Autodesk Inventor part; units mm, degrees
ref_plane "YZ Plane" through (0, 0, 0) normal (1, 0, 0) x (0, 1, 0)
ref_plane "XZ Plane" through (0, 0, 0) normal (0, 1, 0) x (-1, 0, 0)
ref_plane "XY Plane" through (0, 0, 0) normal (0, 0, 1) x (1, 0, 0)
sketch "Sketch2" plane through (0, 0, 0) normal (0, 0, 1) x (1, 0, 0)
  line L0 (0, 0) -> (0, -42.7)
  line L1 (0, 0) -> (-8, 0)
  line L2 (-8, 0) -> (-8, -3.7)
  line L3 (-8, -3.7) -> (0, -3.7)
  line L4 (0, -3.7) -> (0, 0)
  line L5 (0, -3.7) -> (-6, -3.7)
  line L6 (-6, -3.7) -> (-6, -9.7)
  line L7 (-6, -9.7) -> (0, -9.7)
  line L8 (0, -9.7) -> (0, -3.7)
  line L9 (0, -9.7) -> (-8, -9.7)
  line L10 (-8, -9.7) -> (-8, -12.7)
  line L11 (-8, -12.7) -> (0, -12.7)
  line L12 (0, -12.7) -> (0, -9.7)
  line L13 (0, -42.7) -> (-11.15, -42.7)
  line L14 (-11.15, -42.7) -> (-11.15, -41.7)
  line L15 (-11.15, -41.7) -> (0, -41.7)
  line L16 (0, -41.7) -> (0, -42.7)
  line L17 (-11.15, -39.2) -> (0, -39.2)
  line L18 (0, -39.2) -> (0, -40.2)
  line L19 (0, -40.2) -> (-11.15, -40.2)
  line L20 (-11.15, -40.2) -> (-11.15, -39.2)
  line L21 (-11.15, -36.7) -> (0, -36.7)
  line L22 (0, -36.7) -> (0, -37.7)
  line L23 (0, -37.7) -> (-11.15, -37.7)
  line L24 (-11.15, -37.7) -> (-11.15, -36.7)
  line L25 (-11.15, -34.2) -> (0, -34.2)
  line L26 (0, -34.2) -> (0, -35.2)
  line L27 (0, -35.2) -> (-11.15, -35.2)
  line L28 (-11.15, -35.2) -> (-11.15, -34.2)
  line L29 (-11.15, -31.7) -> (0, -31.7)
  line L30 (0, -31.7) -> (0, -32.7)
  line L31 (0, -32.7) -> (-11.15, -32.7)
  line L32 (-11.15, -32.7) -> (-11.15, -31.7)
  line L33 (-11.15, -29.2) -> (0, -29.2)
  line L34 (0, -29.2) -> (0, -30.2)
  line L35 (0, -30.2) -> (-11.15, -30.2)
  line L36 (-11.15, -30.2) -> (-11.15, -29.2)
  line L37 (-11.15, -26.7) -> (0, -26.7)
  line L38 (0, -26.7) -> (0, -27.7)
  line L39 (0, -27.7) -> (-11.15, -27.7)
  line L40 (-11.15, -27.7) -> (-11.15, -26.7)
  line L41 (-11.15, -24.2) -> (0, -24.2)
  line L42 (0, -24.2) -> (0, -25.2)
  line L43 (0, -25.2) -> (-11.15, -25.2)
  line L44 (-11.15, -25.2) -> (-11.15, -24.2)
  line L45 (-11.15, -21.7) -> (0, -21.7)
  line L46 (0, -21.7) -> (0, -22.7)
  line L47 (0, -22.7) -> (-11.15, -22.7)
  line L48 (-11.15, -22.7) -> (-11.15, -21.7)
  line L49 (-11.15, -19.2) -> (0, -19.2)
  line L50 (0, -19.2) -> (0, -20.2)
  line L51 (0, -20.2) -> (-11.15, -20.2)
  line L52 (-11.15, -20.2) -> (-11.15, -19.2)
  line L53 (-11.15, -16.7) -> (0, -16.7)
  line L54 (0, -16.7) -> (0, -17.7)
  line L55 (0, -17.7) -> (-11.15, -17.7)
  line L56 (-11.15, -17.7) -> (-11.15, -16.7)
  line L57 (0, -14.2) -> (-8, -14.2)
  line L58 (-8, -14.2) -> (-8, -15.2)
  line L59 (-8, -15.2) -> (0, -15.2)
  line L60 (0, -15.2) -> (0, -14.2)
  line L61 (0, -12.7) -> (0, -39.2)
  line L62 (-4, -15.2) -> (-4, -16.7)
  line L63 (-4, -14.2) -> (-4, -12.7)
  line L64 (-4, -16.7) -> (-6, -41.7)
  line L65 (-4.2, -17.7) -> (-4.2, -19.2)
  line L66 (-4.4, -21.7) -> (-4.4, -20.2)
  line L67 (-4.6, -24.2) -> (-4.6, -22.7)
  line L68 (-4.8, -26.7) -> (-4.8, -25.2)
  line L69 (-5, -29.2) -> (-5, -27.7)
  line L70 (-5.2, -31.7) -> (-5.2, -30.2)
  line L71 (-5.4, -34.2) -> (-5.4, -32.7)
  line L72 (-5.6, -36.7) -> (-5.6, -35.2)
  line L73 (-5.8, -39.2) -> (-5.8, -37.7)
  line L74 (-6, -41.7) -> (-6, -40.2)
  line L75 (0, -17.7) -> (0, -41.7)
  line L76 (0, -12.7) -> (0, -14.2)
  line L77 (0, -15.2) -> (0, -16.7)
  line L78 (0, -30.2) -> (0, -31.7)
  line L79 (0, -42.7) -> (-2, -42.7)
  line L80 (-2, -42.7) -> (-2, -49.8)
  line L81 (-2, -49.8) -> (0, -49.8)
  line L82 (0, -49.8) -> (0, -42.7)
  line L83 (0, -49.8) -> (-3, -49.8)
  line L84 (-3, -49.8) -> (-3, -55.8)
  line L85 (-3, -55.8) -> (0, -55.8)
  line L86 (0, -55.8) -> (0, -49.8)
  line L87 (0, -55.8) -> (-2.5, -55.8)
  line L88 (-2.5, -55.8) -> (-2.5, -57.3)
  line L89 (-2.5, -57.3) -> (0, -57.3)
  line L90 (0, -57.3) -> (0, -55.8)
  line L91 (0, -57.3) -> (-3.5, -57.3)
  line L92 (-3.5, -57.3) -> (-3.5, -60.3)
  line L93 (-3.5, -60.3) -> (0, -60.3)
  line L94 (0, -60.3) -> (0, -57.3)
  line L95 (-1.9004, -60.3) -> (-0.5, -62.3)
  line L96 (-0.5, -62.3) -> (0, -62.3)
  line L97 (0, -62.3) -> (0, -60.3)
  dimension "d21" = 42.7
  dimension "d22" = 8
  dimension "d23" = 3.7
  dimension "d24" = 6
  dimension "d25" = 6
  dimension "d26" = 8
  dimension "d27" = 3
  dimension "d28" = 11.15
  dimension "d29" = 1
  dimension "d39" = 2.5
  dimension "d44" = 8
  dimension "d45" = 1
  dimension "d46" = 1.5
  dimension "d48" = 12
  dimension "d50" = 2
  dimension "d51" = 7.1
  dimension "d52" = 3
  dimension "d53" = 6
  dimension "d54" = 2.5
  dimension "d55" = 1.5
  dimension "d56" = 3.5
  dimension "d57" = 10.5
  dimension "d58" = 125
  dimension "d59" = 0.5
  dimension "d60" = 2
revolve "Revolution1" add sketch "Sketch2" angle 360 about axis through (0, -31.7, 0) along (0, -1, 0)
sketch "Sketch3" plane through (0, -60.3, 0) normal (0, -1, 0) x (1, 0, 0)
  circle A0 centre (0, 0) radius 3.5
  circle A1 centre (0, 0) radius 1.9004
  line L0 (4.0415, 0) -> (2.0207, -3.5)
  line L1 (2.0207, -3.5) -> (-2.0207, -3.5)
  line L2 (-2.0207, -3.5) -> (-4.0415, 0)
  line L3 (-4.0415, 0) -> (-2.0207, 3.5)
  line L4 (-2.0207, 3.5) -> (2.0207, 3.5)
  line L5 (2.0207, 3.5) -> (4.0415, 0)
  circle A2 centre (0, 0) radius 12.5
  dimension "d61" = 7
  dimension "d62" = 25
extrude "Extrusion1" add sketch "Sketch3" against normal up to surface (3 mm away) contours A0 L5 L0 | A0 L4 L5 | L0 L1 A0 | A0 L3 L4 | L1 L2 A0 | A0 L2 L3
sketch "Sketch4" plane through (0, 0, 0) normal (1, 0, 0) x (0, 1, 0)
  line L0 (-45.05, 15.5) -> (-56.55, 15.5)
  line L1 (-56.55, 15.5) -> (-56.55, -4.5)
  line L2 (-56.55, -4.5) -> (-45.05, -4.5)
  line L3 (-45.05, -4.5) -> (-45.05, 15.5)
  arc A0 (-53.05, 9.9834) -> (-52.05, 9.9834) centre (-52.55, 7) ccw
  line L4 (-60.3, 0) -> (-57.3, 0)
  line L5 (-52.55, 7) -> (-52.55, 15.5) construction
  line L6 (-53.05, 15.5) -> (-53.05, 9.9834)
  line L7 (-52.05, 9.9834) -> (-52.05, 15.5)
  line L8 (-57.3, 2.5) -> (-55.8, 2.5)
  point P0 (0, 0)
  point P1 (-52.55, 11.25)
  point P2 (-56.55, 2.5)
  dimension "d65" = 11.5
  dimension "d66" = 20
  dimension "d67" = 6.05
  dimension "d68" = 4
  dimension "d69" = 11.5
  dimension "d70" = 4.5
  dimension "d84" = 3.5
  dimension "d85" = 4.5
extrude "Extrusion2" add sketch "Sketch4" along normal mid plane 16 contours L3 L2 L1 L0 L6 A0 L7
sketch "Sketch5" plane through (0, -62.3, 0) normal (0, -1, 0) x (1, 0, 0)
  circle A0 centre (0, 0) radius 0.2
  dimension "d75" = 0.4
extrude "Extrusion3" cut sketch "Sketch5" against normal through all
sketch "Sketch6" plane through (0, 0, 0) normal (0, 1, 0) x (1, 0, 0)
  circle A0 centre (0, 0) radius 1
  dimension "d78" = 2
extrude "Extrusion4" cut sketch "Sketch6" against normal up to surface (60.3 mm away)
chamfer "Chamfer1" distance 1 angle 45 1 edges at (-1, 0, 0)
chamfer "Chamfer2" distance 0.5 angle 45 14 edges at (-8, -56.55, 5.5) (0, -56.55, 15.5) (-8, -54.8, 15.5) (-8, -48.55, 15.5) (8, -48.55, 15.5) (0, -45.05, 15.5) (-8, -45.05, 5.5) (-8, -50.8, -4.5) (0, -56.55, -4.5) (8, -56.55, 5.5) (8, -50.8, -4.5) (8, -45.05, 5.5) (8, -54.8, 15.5) (0, -45.05, -4.5)
sketch "Sketch7" plane through (0, 0, 0) normal (0, 0, 1) x (1, 0, 0)
  line L0 (-4.0415, -60.3) -> (-2.0207, -60.3)
  line L1 (-4.0415, -60.3) -> (-4.0415, -57.3)
  line L2 (-4.0415, -60.05) -> (-3.7915, -60.3)
  line L3 (0, -74.76) -> (0, 12.46)
  line L4 (-2.0207, -57.3) -> (-4.0415, -57.3)
  line L5 (-4.0415, -57.55) -> (-3.7915, -57.3)
  point P0 (0, 0)
  dimension "d89" = 0.25
  dimension "d90" = 0.25
  dimension "d92" = 0.25
  dimension "d93" = 0.25
revolve "Revolution2" cut sketch "Sketch7" angle 360 about axis through (0, -10, 0) along (0, 1, 0)
equation "\"d90\" = d89"
equation "\"d92\" = d89"
equation "\"d93\" = d89"
properties part number "e3dv6"
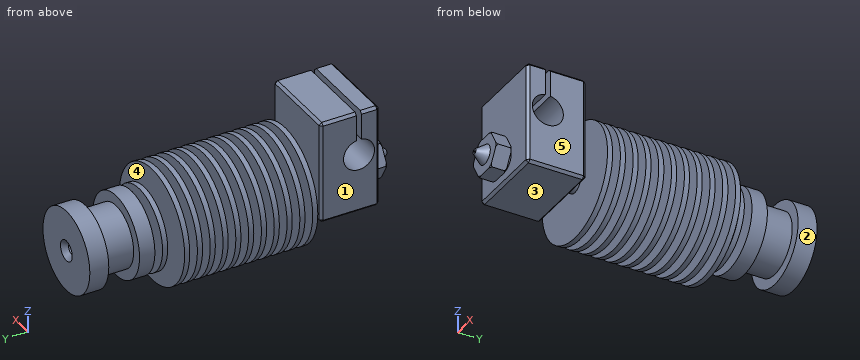
Geometry: final body of the model. Coordinates: model frame, mm. Face numbers are marked on the shaded views. A direction names the side the tool comes from. Round coordinates to 2 decimals unless told otherwise and drop trailing zeros. Order: outer loops, then holes, each group sorted by start corner. A loop starts at its lowest first (then second) coordinate and runs counter-clockwise, first axis right, second up. Notation, with made-up numbers: (37.25, -25) - (94.25, -25) arc R32 ccw to (94.25, 7) - close; hole circle Ø9 at (39, 59.25). An arc over 180 degrees is marked (long way). Write item = value, one per line. Start each with the question number.
Q1. Access query for the marked faces 1, 2, 3, 4 and 5. Directions: +Z, -Z, +X, -X, +Y, -Y. A direction counts if a zero-diameter tool reaches every point of the face in a straight line with its end or side. Return the directions, or none.
Q2. Cut plane B-B on z = 6.75. Give the number of separate pieces and of enclosed holes in the cut face, and give its area (3 significant figures).
Q3. Pin query (flat end, axial travel): pin 1 (12 mm diameter, centred on x = 6, z = -6, fed in from -Y); pin 2 (7.5 mm diameter, centred on x = 3, z = 7, fed in from -Y); pin 3 (1.5 mm diameter, centred on x = -0.5, y = -13.5, fed in from +Z). Return the tip coordinate at first contact, or that it passes through.
Q4. Cut plane A-A on y = -26. Return the cut outline in (x, z), and give its area (3 significant figures).
Q5. Ray query, line 1 (Z direction, x = 0, y = -16); line 2 (Y direction, x = -6.75, z = 11.5); line 3 (X direction, y = -44.5, z = 0). Return the intervals inside material, ascending. Write a range as from..to.
Outcome:
q1.face_1 = +Z, -Z, -X, -Y
q1.face_2 = +Y
q1.face_3 = -Z, +X, -X, -Y
q1.face_4 = none
q1.face_5 = +Z, -Z, +X, -Y
q2.separate_pieces = 16
q2.enclosed_holes = 0
q2.area = 348 mm^2
q3.pin_1 = -60.3
q3.pin_2 = -60.22
q3.pin_3 = 8
q4.outline = circle Ø9.6 at (0, 0); hole circle Ø2 at (0, 0)
q4.area = 69.2 mm^2
q5.line_1 = -4..-1, 1..4
q5.line_2 = -56.55..-53.05, -52.05..-45.05
q5.line_3 = -2..-1, 1..2
